Read the model definition and answer for the solid it produces. Units are mm, in the model's axes. Round coordinates to 2 decimals unless told otherwise and drop trailing zeros. Order: outer loops, then holes, each group sorted by start corner. A loop starts at its lowest first (then second) coordinate and runs counter-clockwise, first axis right, second up. Notation, with made-up numbers: (-5, -6.5) -> (31, -6.5) arc R23 ccw to (31, 9.5) -> close; hole circle Ø9 at (-39, 34.5). An arc over 180 degrees is marked (long way). One line per item, written item: value. Start each with the question number.
1. The mould has two halves that part along Z. Classify faces 1 (the face through (-3, 228, 248)), 2 (the face through (-1.48, 186.12, 104.75)): released by +Z, released by -Z, zero draft, split by the parting line, or undercut.
2. A flat-ended cylindrical pin translates along its axis: pin 1 Ø1 at (x, y) = (-2.5, 303.5) entering from -Z. Find the tip coordinate at first contact, or state that the pin passes through.
3. Section C-C (x = -2.4) is taken. State how many separate pieces and enclosed holes the cut face has, then the cut area to 3 significant figures.
4. Section B-B (z = 373.5) is taken. Give the vertices of the cut face in (x, y).
5. Section A-A (y = 55) is taken. Give the vertices of the cut face in (x, z), then the cut area to 3 significant figures.
6. Consider line 1 (Z direction, x = -0.35, y = 370.5); line 2 (Y direction, x = -1.5, z = 376); line 3 (Z direction, x = -0.9, y = 165). Determine where each line is inside the solid, lowest interval first.
from build123d import *

# Parameters (mm, degrees)
PAD_DEPTH    = 3
SKETCH003_R  = 25
POCKET_DEPTH = 3.001


with BuildPart() as part:
    # Sketch → Pad (new body)
    with BuildSketch(Plane.YZ):
        Polygon((0, 0), (0, 490), (450, 490), (450, 0), (225, 0), align=None)
    extrude(amount=-PAD_DEPTH)

    # Sketch003 → Pocket (cut, through all)
    with BuildSketch(Plane.YZ):
        with Locations((372.684972, 383.665641)):
            Circle(SKETCH003_R)
        with Locations((272.684972, 383.665641)):
            Circle(SKETCH003_R)
        with Locations((72.684972, 383.665641)):
            Circle(SKETCH003_R)
        with Locations((72.684972, 83.665641)):
            Circle(SKETCH003_R)
        with Locations((172.684972, 83.665641)):
            Circle(SKETCH003_R)
        with Locations((372.684972, 83.665641)):
            Circle(SKETCH003_R)
        with Locations((272.684972, 83.665641)):
            Circle(SKETCH003_R)
        with Locations((172.684972, 383.665641)):
            Circle(SKETCH003_R)
    extrude(amount=-POCKET_DEPTH, mode=Mode.SUBTRACT)


solid = part.part
Answer:
1. face 1: zero draft
1. face 2: undercut
2. pin 1: z = 0
3. separate pieces: 1
3. enclosed holes: 8
3. area: 205,000 mm^2
4. outline: (-3, 0) -> (0, 0) -> (0, 49.85) -> (-3, 49.85) -> close; (-3, 95.52) -> (0, 95.52) -> (0, 149.85) -> (-3, 149.85) -> close; (-3, 195.52) -> (0, 195.52) -> (0, 249.85) -> (-3, 249.85) -> close; (-3, 295.52) -> (0, 295.52) -> (0, 349.85) -> (-3, 349.85) -> close; (-3, 395.52) -> (0, 395.52) -> (0, 450) -> (-3, 450) -> close
5. outline: (-3, 0) -> (0, 0) -> (0, 66) -> (-3, 66) -> close; (-3, 101.34) -> (0, 101.34) -> (0, 366) -> (-3, 366) -> close; (-3, 401.34) -> (0, 401.34) -> (0, 490) -> (-3, 490) -> close
5. area: 1,260 mm^2
6. line 1: 0 to 58.76, 108.57 to 358.76, 408.57 to 490
6. line 2: 0 to 48.89, 96.48 to 148.89, 196.48 to 248.89, 296.48 to 348.89, 396.48 to 450
6. line 3: 0 to 59.88, 107.46 to 359.88, 407.46 to 490
